Autodesk Inventor part; units mm, degrees
ref_plane "YZ Plane" through (0, 0, 0) normal (1, 0, 0) x (0, 1, 0)
ref_plane "XZ Plane" through (0, 0, 0) normal (0, 1, 0) x (-1, 0, 0)
ref_plane "XY Plane" through (0, 0, 0) normal (0, 0, 1) x (1, 0, 0)
sketch "Sketch1" plane through (0, 0, 0) normal (0, 0, 1) x (1, 0, 0)
  line L0 (1.4434, -2.5) -> (-1.4434, -2.5)
  line L1 (-1.4434, -2.5) -> (-2.8868, 0)
  line L2 (-2.8868, 0) -> (-1.4434, 2.5)
  line L3 (-1.4434, 2.5) -> (1.4434, 2.5)
  line L4 (1.4434, 2.5) -> (2.8868, 0)
  line L5 (2.8868, 0) -> (1.4434, -2.5)
  point P0 (0, 0)
  point P1 (0, 0)
  dimension "d0" = 5
extrude "Extrusion1" add sketch "Sketch1" against normal blind 5
sketch "Sketch2" plane through (0, 0, 0) normal (0, 0, 1) x (1, 0, 0)
  circle A0 centre (0, 0) radius 1.25
  dimension "d3" = 2.5
extrude "Extrusion2" cut sketch "Sketch2" against normal blind 3
sketch "Sketch3" plane through (0, 0, -5) normal (0, 0, -1) x (-1, 0, 0)
  circle A0 centre (0, 0) radius 1.25
  dimension "d6" = 2.5
extrude "Extrusion3" add sketch "Sketch3" along normal blind 6
thread "Thread1"
thread "Thread2"
fillet "Fillet1" radius 0.2 12 edges at (0, -2.5, -5) (-2.1651, -1.25, -5) (-2.1651, 1.25, -5) (0, 2.5, -5) (2.1651, 1.25, -5) (2.1651, -1.25, -5) (0, -2.5, 0) (2.1651, -1.25, 0) (2.1651, 1.25, 0) (0, 2.5, 0) (-2.1651, 1.25, 0) (-2.1651, -1.25, 0)
fillet "Fillet1" radius 0.2 6 edges at (-2.8868, 0, -2.5) (-1.4434, 2.5, -2.5) (1.4434, 2.5, -2.5) (2.8868, 0, -2.5) (1.4434, -2.5, -2.5) (-1.4434, -2.5, -2.5)
equation "\"d0\" = m3hs_hexDiam"
equation "\"d1\" = m3hs_bodyLength"
equation "\"d3\" = m3hs_threadDiam"
equation "\"d4\" = m3hs_holeDepth"
equation "\"d6\" = m3hs_threadDiam"
equation "\"d7\" = m3hs_studLength"
equation "\"d13\" = m3hs_rounding"
equation "\"m3hs_hexDiam\" = 5"
equation "\"m3hs_bodyLength\" = 5"
equation "\"m3hs_holeDepth\" = 3"
equation "\"m3hs_studLength\" = 6"
equation "\"m3hs_rounding\" = 0.2"
equation "\"m3hs_threadDiam\" = 2.5"
properties part number "M2.5 Hex Spacer 5mm" material "Stainless Steel"
Check sheet for the modelled part. Datum: model origin and axes. Units: mm. A direction names the side the tool comes from. Round coordinates to 2 decimals unless told otherwise and drop trailing zeros. Order: outer loops, then holes, each group sorted by start corner. A loop starts at its lowest first (then second) coordinate and runs counter-clockwise, first axis right, second up. Notation, with made-up numbers: (38.5, -29) -> (70.5, -29) arc R20 cw to (70.5, -21) -> close; hole circle Ø7 at (45.5, 86). An arc over 180 degrees is marked (long way). One line per item, written item: value. Start each with the question number.
Q1. Cross-section at C-C (z = -4). Record the boundary of the cut face in (x, y).
Q2. Cross-section at B-B (x = 0). Record the boundary of the cut face in (y, z).
Q3. Set-up check for faces 1 (the face through (1, 1, -5)), 2 (the face through (-2.104, 1.236, -4.943)): record each of +Z, -Z, +X, -X, +Y, -Y from which the full face is reachable in a straight line by a thin tool's end or side.
Q4. Cross-section at A-A (z = -1.25). Record the boundary of the cut face in (x, y), and give its area (3 significant figures).
Q5. Thickness scan on line 1 (Y direction, x = 0, z = -0.55); line 2 (Z direction, x = -1.85, y = 0.5); line 3 (Y direction, x = -1.5, z = -2.25). Record the ranges inside material, lowest first.
Q6. Gauge pin test, flat ends, axial feed: pin 1 Ø1 at (y, z) = (-1.5, -1.5) entering from +X; pin 2 Ø1 at (y, z) = (-2, -7) entering from +X. Record the tip position at first contact, or that the pin passes through.
Q7. Mould release check, pull along X, two halves, no side actions. Record for faces 3 (the face through (-2.174, 1.234, -2.468)), 4 (the face through (0, 0, -3)), 5 (the face through (2.122, 1.204, -4.943)): pulls with the +X half, pulls with the -X half, needs draft (parallel to the pull), parting line crosses it, or undercut.
Completed:
1. outline: (-2.83, -0.1) -> (-1.5, -2.4) arc R0.2 ccw to (-1.33, -2.5) -> (1.33, -2.5) arc R0.2 ccw to (1.5, -2.4) -> (2.83, -0.1) arc R0.2 ccw to (2.83, 0.1) -> (1.5, 2.4) arc R0.2 ccw to (1.33, 2.5) -> (-1.33, 2.5) arc R0.2 ccw to (-1.5, 2.4) -> (-2.83, 0.1) arc R0.2 ccw to start
2. outline: (-2.5, -4.8) arc R0.2 ccw to (-2.3, -5) -> (-1.25, -5) -> (-1.25, -11) -> (1.25, -11) -> (1.25, -5) -> (2.3, -5) arc R0.2 ccw to (2.5, -4.8) -> (2.5, -0.2) arc R0.2 ccw to (2.3, 0) -> (1.25, 0) -> (1.25, -3) -> (-1.25, -3) -> (-1.25, 0) -> (-2.3, 0) arc R0.2 ccw to (-2.5, -0.2) -> close
3. face 1: -Z
3. face 2: -Z, -X, +Y
4. outline: (-2.83, -0.1) -> (-1.5, -2.4) arc R0.2 ccw to (-1.33, -2.5) -> (1.33, -2.5) arc R0.2 ccw to (1.5, -2.4) -> (2.83, -0.1) arc R0.2 ccw to (2.83, 0.1) -> (1.5, 2.4) arc R0.2 ccw to (1.33, 2.5) -> (-1.33, 2.5) arc R0.2 ccw to (-1.5, 2.4) -> (-2.83, 0.1) arc R0.2 ccw to start; hole circle Ø2.5 at (0, 0)
4. area: 16.7 mm²
5. line 1: y = -2.5 to -1.25, 1.25 to 2.5
5. line 2: z = -5 to 0
5. line 3: y = -2.4 to 2.4
6. pin 1: stops at x = 2.31
6. pin 2: passes through
7. face 3: pulls with the -X half
7. face 4: undercut
7. face 5: pulls with the +X half
